```python
from build123d import *

# Parameters (mm, degrees)
SKETCH1_W           = 54.8
SKETCH1_H           = 54.8
SKETCH1_W_2         = 50.8
SKETCH1_H_2         = 50.8
BOSS_EXTRUDE1_DEPTH = 2
SKETCH2_W           = 54.8
SKETCH2_H           = 54.8
SKETCH2_W_2         = 50.8
SKETCH2_H_2         = 50.8
BOSS_EXTRUDE2_DEPTH = 5
FILLET1_R           = 2


with BuildPart() as part:
    # Sketch1 → Boss-Extrude1 (new body)
    # profile 1 of 2: a face of its own
    with BuildSketch(Plane.XY):
        Rectangle(SKETCH1_W, SKETCH1_H)
        Rectangle(SKETCH1_W_2, SKETCH1_H_2, mode=Mode.SUBTRACT)
    # profile 2 of 2: a face of its own
    with BuildSketch(Plane.XY):
        Rectangle(SKETCH1_W_2, SKETCH1_H_2)
    extrude(amount=BOSS_EXTRUDE1_DEPTH)

    # Sketch2 → Boss-Extrude2 (add)
    with BuildSketch(Plane.XY.offset(2)):
        Rectangle(SKETCH2_W, SKETCH2_H)
        Rectangle(SKETCH2_W_2, SKETCH2_H_2, mode=Mode.SUBTRACT)
    extrude(amount=BOSS_EXTRUDE2_DEPTH)

    # Fillet1
    fillet1_edges = [part.edges().sort_by_distance(p)[0] for p in [
        (-25.4, -25.4, 4.5),
        (25.4, -25.4, 4.5),
        (25.4, 25.4, 4.5),
        (-25.4, 25.4, 4.5),
        (27.4, 27.4, 3.5),
        (27.4, -27.4, 3.5),
        (-27.4, -27.4, 3.5),
        (-27.4, 27.4, 3.5),
    ]]
    fillet(fillet1_edges, radius=FILLET1_R)


solid = part.part
```
For this review, take the finished solid that the model builds, in its own axes (mm). A direction names the side the tool comes from. Round coordinates to 2 decimals unless told otherwise and drop trailing zeros. Loops run counter-clockwise (first coordinate to the right, second up) from the corner with the lowest first, then second, coordinate; pieces in that order, holes last.
Q1. Add section B-B on y = -20. Write out the cut boundary in (x, z).
Result sheet:
outline: (-27.4, 0) - (27.4, 0) - (27.4, 7) - (25.4, 7) - (25.4, 2) - (-25.4, 2) - (-25.4, 7) - (-27.4, 7) - close
Q2. Mouldability with a two-part tool opening along X and no side actions: class faces 1 (the face through (26.8, -26.83, 3.55)), 2 (the face through (-27.4, 0, 3)), 3 (the face through (0, 0, 0)), 4 (the face through (24.8, 24.83, 4.54)) as +X half, -X half, draft (parallel to the pull), parting line (faces both ways), or undercut.
Result sheet:
face 1: +X half
face 2: -X half
face 3: draft
face 4: undercut
Q3. Insertion check: pin 1 Ø5 at (x, y) = (-15, -14.5) entering from +Z. The pin has a flat end and moves straight along its axis. Give the tip position at first contact, or say it passes through.
Result sheet:
pin 1: stops at z = 2
Q4. To check wall thickness, follow line 1 along Y through (x, z) = (15, 6.5); line 2 along Z through (x, y) = (5, -7). State the ranges of each line that lie inside material, in increasing order.
Result sheet:
line 1: y = -27.4 to -25.4, 25.4 to 27.4
line 2: z = 0 to 2
Q5. Machinability: for faces 5 (the face through (0, 25.4, 4)), 6 (the face through (26.83, 26.8, 3.45)), which of the approach directions +Z, -Z, +X, -X, +Y, -Y give a long, thin tool a straight path to every point of the face, cutting with its end or side? Answer none if there is none.
Result sheet:
face 5: +Z
face 6: +Z, -Z, +X, +Y
Q6. Add section A-A on z = 3.75. Write out the cut boundary in (x, y).
Result sheet:
outline: (-27.4, -25.4) arc R2 ccw to (-25.4, -27.4) - (25.4, -27.4) arc R2 ccw to (27.4, -25.4) - (27.4, 25.4) arc R2 ccw to (25.4, 27.4) - (-25.4, 27.4) arc R2 ccw to (-27.4, 25.4) - close; hole (-25.4, -23.4) arc R2 ccw to (-23.4, -25.4) - (23.4, -25.4) arc R2 ccw to (25.4, -23.4) - (25.4, 23.4) arc R2 ccw to (23.4, 25.4) - (-23.4, 25.4) arc R2 ccw to (-25.4, 23.4) - close
